from build123d import *

# Parameters (mm, degrees)
F0_W           = 200
F0_H           = 100
F1_DEPTH       = 30
F2_D           = 15
F2_CSINK_D     = 20
F2_CSINK_ANGLE = 90
F3_D           = 30
F3_CSINK_D     = 40
F3_CSINK_ANGLE = 90
F4_D           = 45
F4_CSINK_D     = 55
F4_CSINK_ANGLE = 90
F5_SIZE        = 10


with BuildPart() as f1:
    # F0 (on Top) → F1 (new body)
    with BuildSketch(Plane.XY):
        with Locations((100, 50)):
            Rectangle(F0_W, F0_H)
    extrude(amount=-F1_DEPTH)

    # F2 (through all)
    with Locations(Plane.XY):
        with Locations((25, 50.437499)):
            CounterSinkHole(F2_D / 2, F2_CSINK_D / 2, counter_sink_angle=F2_CSINK_ANGLE)

    # F3 (through all)
    with Locations(Plane.XY):
        with Locations((75, 50.437499)):
            CounterSinkHole(F3_D / 2, F3_CSINK_D / 2, counter_sink_angle=F3_CSINK_ANGLE)

    # F4 (through all)
    with Locations(Plane.XY):
        with Locations((150, 50.437499)):
            CounterSinkHole(F4_D / 2, F4_CSINK_D / 2, counter_sink_angle=F4_CSINK_ANGLE)

    # F5
    f5_edges = [f1.edges().sort_by_distance(p)[0] for p in [
        (200, 50, 0),
        (200, 50, -30),
        (0, 50, 0),
        (0, 50, -30),
        (100, 100, 0),
        (100, 100, -30),
        (100, 0, 0),
        (100, 0, -30),
    ]]
    chamfer(f5_edges, length=F5_SIZE)


solid = f1.part
Read the model definition and answer for the solid it produces. Units are mm, in the model's axes. Round coordinates to 2 decimals unless told otherwise and drop trailing zeros. Write each loop counter-clockwise with the first axis right and the second up, starting at its lowest first coordinate (ties: lowest second). Pieces come first, ordered by that corner, then holes. Notation, with made-up numbers: (74, -4.75) - (84, -4.75) arc R27 cw to (84, 25.25) - close; hole circle Ø4 at (68, -33.75). An arc over 180 degrees is marked (long way). One line per question, with ' | ' between items. Start each with the question number.
1. Section D-D (y = 20.5) is taken. Determine the outline of the cut face in (x, z).
2. Section A-A (x = 75) is taken. Determine the outline of the cut face in (y, z), and give its area (4 significant figures).
3. Section B-B (x = 150) is taken. Determine the outline of the cut face in (y, z), and give its area (4 significant figures).
4. For a pull along X with two mould halves and no side action, classify faces 1 (the face through (76.98, 65.55, -4.76)), 2 (the face through (99, 95, -25)), 3 (the face through (5, 49, -25)) as +X half, -X half, draft (parallel to the pull), parting line (faces both ways), or undercut.
5. Find the intervals of material crossed by probe 1 along Y at (x, z) = (75, -18); probe 2 along X at (y, z) = (44, -9.25); probe 3 along Y at (x, z) = (25, -19.75), in increasing order. Write a range as [from, to].
6. Each of these flat-tipped pins is pushed along its axis until it touches: pin 1 (12 mm diameter, centred on x = 122, z = -26.5, fed in from -Y); pin 2 (5 mm diameter, centred on y = 61.5, z = -24.5, fed in from -X). Where does it stop, or does it pass through?
7. Section C-C (z = -27) is taken. Determine the outline of the cut face in (x, y).
Filled in:
1) outline: (0, -20) - (10, -30) - (190, -30) - (200, -20) - (200, -10) - (190, 0) - (10, 0) - (0, -10) - close
2) outline: (0, -20) - (10, -30) - (35.44, -30) - (35.44, -5) - (30.44, 0) - (10, 0) - (0, -10) - close; (65.44, -30) - (90, -30) - (100, -20) - (100, -10) - (90, 0) - (70.44, 0) - (65.44, -5) - close | area: 1,875 mm²
3) outline: (0, -20) - (10, -30) - (27.94, -30) - (27.94, -5) - (22.94, 0) - (10, 0) - (0, -10) - close; (72.94, -30) - (90, -30) - (100, -20) - (100, -10) - (90, 0) - (77.94, 0) - (72.94, -5) - close | area: 1,425 mm²
4) face 1: undercut | face 2: draft | face 3: -X half
5) probe 1: [0, 35.44], [65.44, 100] | probe 2: [0.75, 21.15], [28.85, 61.45], [88.55, 128.44], [171.56, 199.25] | probe 3: [0, 42.94], [57.94, 100]
6) pin 1: y = 0.5 | pin 2: x = 2
7) outline: (7, 7) - (193, 7) - (193, 93) - (7, 93) - close; hole circle Ø15 at (25, 50.44); hole circle Ø30 at (75, 50.44); hole circle Ø45 at (150, 50.44)
